Job drawing, mm, ordinate dimensions from the low corner. One solid piece. Round coordinates to 2 decimals unless told otherwise and drop trailing zeros. Loops run counter-clockwise (first coordinate to the right, second up) from the corner with the lowest first, then second, coordinate; pieces in that order, holes last.
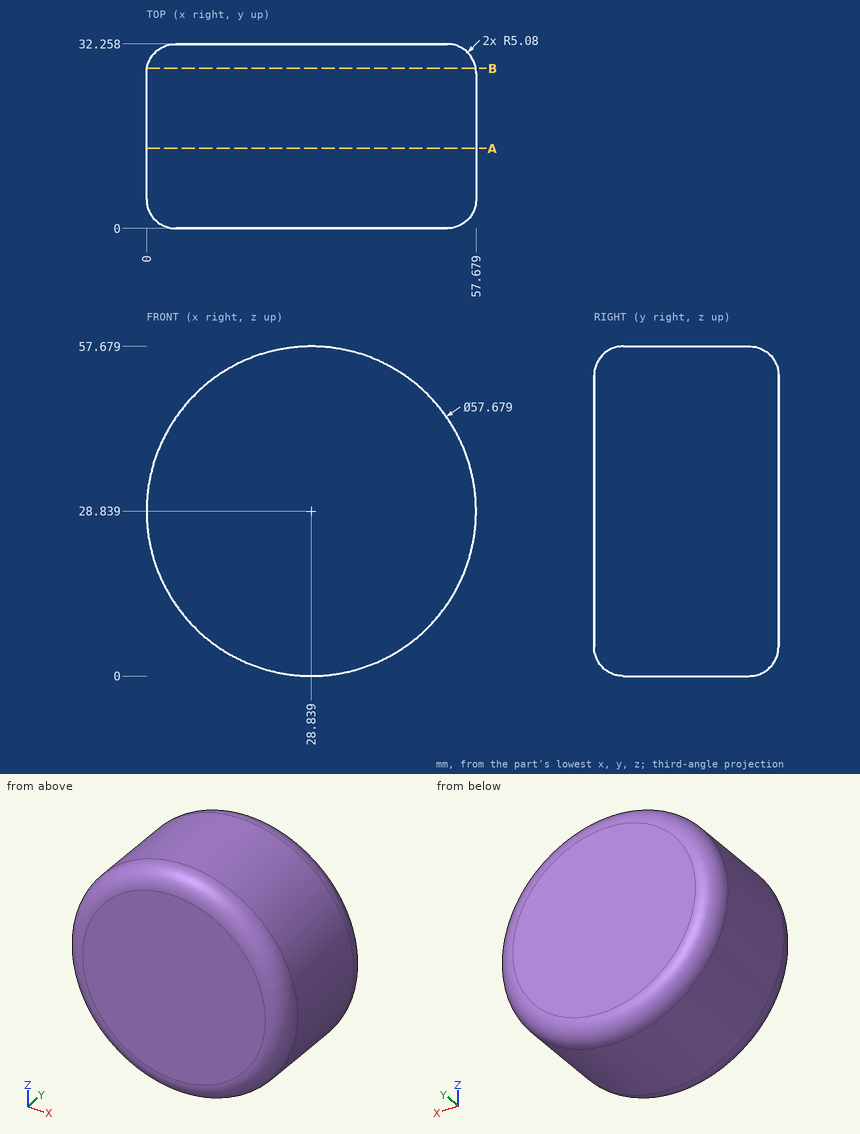
(1) Slice it at A-A on y = 14. List the corners of the cut face in (x, z), plus the area to 3 significant figures.
Responses:
outline: circle Ø57.68 at (28.84, 28.84)
area: 2,610 mm2
(2) Probe line 1 (X direction, y = 19, z = 29); line 2 (Z direction, x = 4.5, y = 11.5) (1 decimal); line 3 (Z direction, x = 37.5, y = 9.5). List the from-to ranges inside material, lowest first.
Responses:
line 1: x = 0 to 57.68
line 2: z = 13.4 to 44.3
line 3: z = 1.33 to 56.35
(3) Slice it at B-B on y = 28. List the corners of the cut face in (x, z) (1 decimal), plus the area to 3 significant figures.
Responses:
outline: circle Ø57.5 at (28.8, 28.8)
area: 2,600 mm2
(4) Pin check, flat tips, straight feed: P1, Ø8, axis at x = 12.5, z = 28, coming from the -Y side; P2, Ø12, axis at x = 8.5, y = 20, coming from the -Z side; P3, Ø4, axis at y = 3.5, z = 37, coming from the -X side; P4, Ø4, axis at x = 8, y = 27, coming from the -Z side (1 decimal). Stop position of each tip, or through.
Responses:
P1: stops at y = 0
P2: stops at z = 3.82
P3: stops at x = 0.76
P4: stops at z = 7
